Geometry: see drawing. Coordinates: mm, zero at the bounding-box minimum. Coordinates: 2 decimals unless noted, no trailing zeros. Loops run counter-clockwise (first coordinate to the right, second up) from the corner with the lowest first, then second, coordinate; pieces in that order, holes last. Notation, with made-up numbers: (55.25, 84.25) -> (88.25, 84.25) arc R13 ccw to (88.25, 90.25) -> close; hole circle Ø6 at (48, -9.75). An arc over 180 degrees is marked (long way). One line per item, written item: value. Start each with the question number.
Item 1: Section query A-A on z = 39. Return loops of the section in (x, y) (1 decimal).
Item 2: Section query D-D on x = 32. Return loops of the section in (y, z) (1 decimal), then the cut area to 3 significant figures.
Item 3: Section query C-C on x = 10.5. Return loops of the section in (y, z).
Item 4: Section query B-B on y = 11. Return loops of the section in (x, z) (1 decimal), then the cut area to 3 significant figures.
Item 5: Ray query, probe 1 along Y at (x, z) = (12, 72); probe 2 along X at (y, z) = (6, 12.5) (1 decimal); probe 3 along X at (y, z) = (10, 30.5) (1 decimal). Return the intervals inside material, ascending. Write a range as from..to.
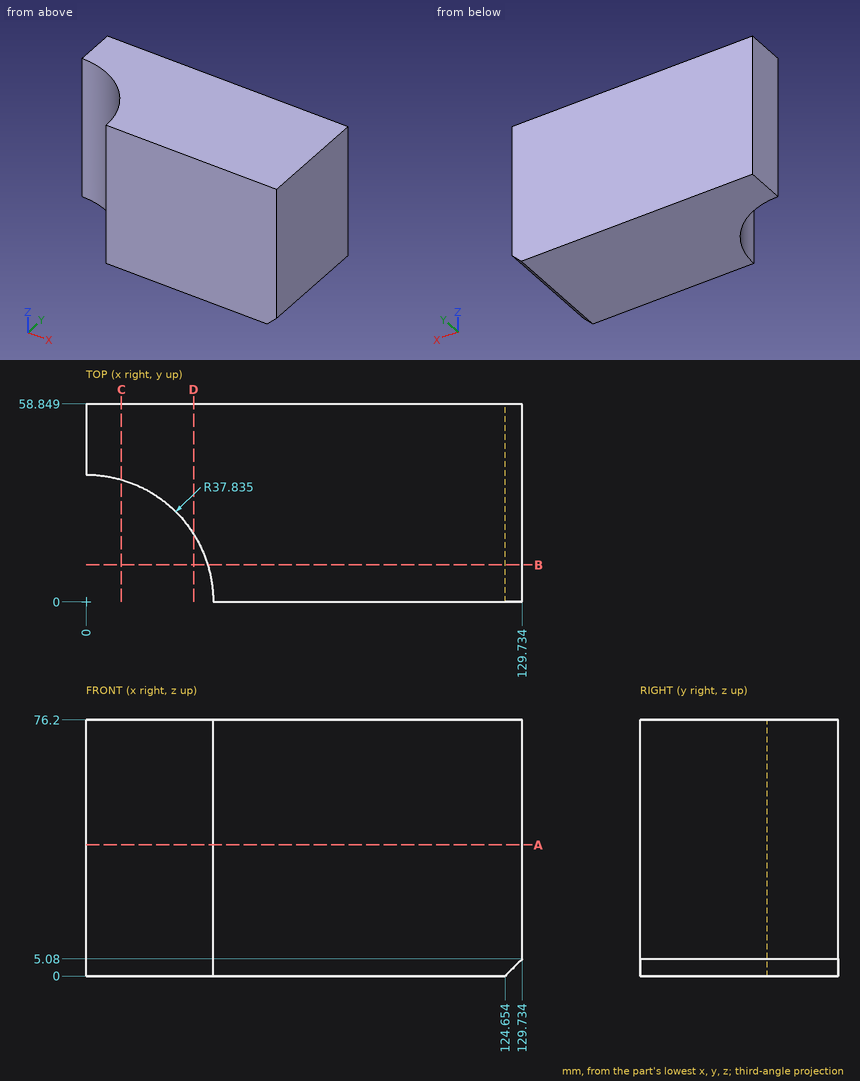
Reply:
1. outline: (0, 37.8) arc R37.8 cw to (37.8, 0) -> (129.7, 0) -> (129.7, 58.8) -> (0, 58.8) -> close
2. outline: (20.2, 0) -> (58.8, 0) -> (58.8, 76.2) -> (20.2, 76.2) -> close
2. area: 2,950 mm²
3. outline: (36.35, 0) -> (58.85, 0) -> (58.85, 76.2) -> (36.35, 76.2) -> close
4. outline: (36.2, 0) -> (124.7, 0) -> (129.7, 5.1) -> (129.7, 76.2) -> (36.2, 76.2) -> close
4. area: 7,110 mm²
5. probe 1: y = 35.88..58.85
5. probe 2: x = 37.4..129.7
5. probe 3: x = 36.5..129.7
